```python
from build123d import *

# Parameters (mm, degrees)
F0_R     = 1.5
F1_DEPTH = 47.3
F2_R     = 11
F2_R_2   = 4
F3_DEPTH = 2
F4_R     = 2.5
F5_DEPTH = 24


with BuildPart() as f1:
    # F0 (on Top) → F1 (new body)
    with BuildSketch(Plane.XY):
        with BuildLine():
            Line((16.1, 21.1), (-16.1, 21.1))
            ThreePointArc((-16.1, 21.1), (-19.635534, 19.635534), (-21.1, 16.1))
            Line((-21.1, 16.1), (-21.1, -16.1))
            ThreePointArc((-21.1, -16.1), (-19.635534, -19.635534), (-16.1, -21.1))
            Line((-16.1, -21.1), (16.1, -21.1))
            ThreePointArc((16.1, -21.1), (19.635534, -19.635534), (21.1, -16.1))
            Line((21.1, -16.1), (21.1, 16.1))
            ThreePointArc((21.1, 16.1), (19.635534, 19.635534), (16.1, 21.1))
        make_face()
        with Locations((-15.52, -15.52)):
            Circle(F0_R, mode=Mode.SUBTRACT)
        with Locations((15.52, -15.52)):
            Circle(F0_R, mode=Mode.SUBTRACT)
        with Locations((-15.52, 15.52)):
            Circle(F0_R, mode=Mode.SUBTRACT)
        with Locations((15.52, 15.52)):
            Circle(F0_R, mode=Mode.SUBTRACT)
    extrude(amount=F1_DEPTH)

    # F2 (on face) → F3 (join)
    with BuildSketch(Plane.XY.offset(47.3)):
        Circle(F2_R)
        Circle(F2_R_2, mode=Mode.SUBTRACT)
    extrude(amount=F3_DEPTH)

    # F4 (on face) → F5 (join)
    with BuildSketch(Plane.XY.offset(47.3)):
        Circle(F4_R)
    extrude(amount=F5_DEPTH)


solid = f1.part
```
Design review of the part built by this model. Coordinates are the model's own, in mm. A direction names the side the tool comes from. Give positions to 0.01 mm unless a question says otherwise; leave off trailing zeros. Loops run counter-clockwise (first coordinate to the right, second up) from the corner with the lowest first, then second, coordinate; pieces in that order, holes last. Notation, with made-up numbers: M 78.25,-9.5 L 117.25,-9.5 A25 cw 117.25,6.5 Z; hole C -14,-10 d11. An arc over 180 degrees is marked long. Return JSON: item names as keys, results as strings. Group by question number.
Item 1: We need section D-D (x = -15). Give the boundary of the cut face in (y, z).
Item 2: We need section C-C (z = 43). Give the boundary of the cut face in (x, y).
Item 3: Insertion check: pin 1 Ø1.8 at (x, y) = (-15.52, -15.52) entering from +Z; pin 2 Ø8 at (x, z) = (-2, 61.5) entering from -Y; pin 3 Ø1 at (x, y) = (-8, 10) entering from +Z. Each pin has a flat end and moves straight along its axis. Give the tip position at first contact, or say it passes through.
Item 4: Tool access review of faces 4 (the cylindrical face through (-19.67, -19.6, 23.32)), 5 (the cylindrical face through (-0.867, -3.905, 48.286)): name each direction out of +Z, -Z, +X, -X, +Y, -Y from which nothing blocks a thin tool from reaching the whole face with its end or side.
Item 5: For probe 1 along Y at (x, z) = (-15.52, 12); probe 2 along Y at (x, z) = (0, 47.8); probe 3 along Z at (x, y) = (-8, 16.5), list the stretches that pass through material, from the lowest coordinate up.
Item 6: We need section A-A (y = 0). Give the boundary of the cut face in (x, z), and give its area (3 significant figures).
Item 7: Mouldability with a two-part tool opening along X and no side actions: class faces 1 (the flat face through (0, 0, 71.3)), 2 (the cylindrical face through (-17.02, -15.45, 23.32)), 3 (the cylindrical face through (19.67, 19.6, 23.32)) as released by +X, released by -X, zero draft, split by the parting line, or undercut.
Output:
{
 "1": {"outline": "M -21.1,0 L -16.93,0 L -16.93,47.3 L -21.1,47.3 Z; M -14.11,0 L 14.11,0 L 14.11,47.3 L -14.11,47.3 Z; M 16.93,0 L 21.1,0 L 21.1,47.3 L 16.93,47.3 Z"},
 "2": {"outline": "M -21.1,-16.1 A5 ccw -16.1,-21.1 L 16.1,-21.1 A5 ccw 21.1,-16.1 L 21.1,16.1 A5 ccw 16.1,21.1 L -16.1,21.1 A5 ccw -21.1,16.1 Z; hole C -15.52,-15.52 d3; hole C -15.52,15.52 d3; hole C 15.52,-15.52 d3; hole C 15.52,15.52 d3"},
 "3": {"pin 1": "passes through", "pin 2": "stops at y = -2.5", "pin 3": "stops at z = 47.3"},
 "4": {"face 4": "+Z, -Z, -X, -Y", "face 5": "+Z"},
 "5": {"probe 1": "y = -21.1 to -17.02, -14.02 to 14.02, 17.02 to 21.1", "probe 2": "y = -11 to -4, -2.5 to 2.5, 4 to 11", "probe 3": "z = 0 to 47.3"},
 "6": {"outline": "M -21.1,0 L 21.1,0 L 21.1,47.3 L 11,47.3 L 11,49.3 L 4,49.3 L 4,47.3 L 2.5,47.3 L 2.5,71.3 L -2.5,71.3 L -2.5,47.3 L -4,47.3 L -4,49.3 L -11,49.3 L -11,47.3 L -21.1,47.3 Z", "area": "2,140 mm^2"},
 "7": {"face 1": "zero draft", "face 2": "undercut", "face 3": "released by +X"}
}
